Part model, mm, in its own coordinate system. A direction names the side the tool comes from. Coordinates: 2 decimals unless noted, no trailing zeros. Loops run counter-clockwise (first coordinate to the right, second up) from the corner with the lowest first, then second, coordinate; pieces in that order, holes last. Notation, with made-up numbers: (56, 6.25) -> (110, 6.25) arc R10 cw to (110, 11.25) -> close; hole circle Ø6 at (-30, 45.25). An arc over 180 degrees is marked (long way). One line per question, with ' | ' between items. Start each with the question number.
1) Cut at D-D (z = 30). List the corners of the cut face in (x, y), plus the area to 3 significant figures.
2) Two-plate mould, pull along Z, no slides. Class faces 1 (the face through (5, 5, 0)), 2 (the face through (9, 17, -9)), 3 (the face through (-0.88, 10.92, 19.98)): released by +Z, released by -Z, zero draft, split by the parting line, or undercut.
3) Drop flat-ended pins along their axis: pin 1 (12.5 mm diameter, centred on x = 0.5, z = -5, fed in from +Y); pin 2 (6 mm diameter, centred on y = 4, z = 29.5, fed in from +X); pin 3 (10 mm diameter, centred on x = 12.5, y = 3.5, fed in from +Z). Give the stop position or say it passes through.
4) Probe L1, parallel to X at y = 3.6, z = 0; L2, parallel to X at y = 13.5, z = 0; L3, parallel to Y at x = 32, z = -12. List the from-to ranges inside material, lowest first. Write a range as from..to.
5) 3-axis set-ups, long thin cutter, end or side, ignore diameter. For faces 4 (the face through (25.85, 2.46, 0.92)), 5 (the face through (-18.3, 5, -9.4)): which of +Z, -Z, +X, -X, +Y, -Y reach the whole face in a straight line?
6) Cut at A-A (x = 0). List the corners of the cut face in (y, z), plus the area to 3 significant figures.
7) Cut at B-B (z = 0). List the corners of the cut face in (x, y), plus the area to 3 significant figures.
8) Cut at C-C (y = 2.25). List the corners of the cut face in (x, z), plus the area to 3 significant figures.
from build123d import *

# Parameters (mm, degrees)
SKETCH2_R          = 4.25
CUT_EXTRUDE1_DEPTH = 10


with BuildPart() as part:
    # Sketch1 → Revolve1 (revolve)
    with BuildSketch(Plane.XY, mode=Mode.PRIVATE) as revolve1_sk:
        Polygon((4.5, 5), (12.5, 5), (12.5, 17), (20, 17), (20, 5), (40, 5), (40, 0), (4.5, 0), align=None)
    revolve(revolve1_sk.sketch.rotate(Axis((0, 0, 0), (0, 1, 0)), 90), axis=Axis((0, 0, 0), (0, 1, 0)))

    # Sketch2 → Cut-Extrude1 (cut)
    with BuildSketch(Plane.XZ):
        with Locations(Location((0, 30, 0), (0, 0, 270))):
            Circle(SKETCH2_R)
        with Locations(Location((30, 0, 0), (0, 0, 270))):
            Circle(SKETCH2_R)
        with Locations(Location((0, -30, 0), (0, 0, 270))):
            Circle(SKETCH2_R)
        with Locations(Location((-30, 0, 0), (0, 0, 270))):
            Circle(SKETCH2_R)
    extrude(amount=-CUT_EXTRUDE1_DEPTH, mode=Mode.SUBTRACT)


solid = part.part
Reported:
1) outline: (-26.46, 0) -> (-4.25, 0) -> (-4.25, 5) -> (-26.46, 5) -> close; (4.25, 0) -> (26.46, 0) -> (26.46, 5) -> (4.25, 5) -> close | area: 222 mm²
2) face 1: undercut | face 2: zero draft | face 3: split by the parting line
3) pin 1: stops at y = 5 | pin 2: stops at x = 29.96 | pin 3: stops at z = 39.29
4) L1: x = -40..-34.25, -25.75..-4.5, 4.5..25.75, 34.25..40 | L2: x = -20..-12.5, 12.5..20 | L3: y = 0..5
5) face 4: +Y, -Y | face 5: +Y
6) outline: (0, -40) -> (5, -40) -> (5, -34.25) -> (0, -34.25) -> close; (0, -25.75) -> (5, -25.75) -> (5, -20) -> (17, -20) -> (17, -12.5) -> (5, -12.5) -> (5, -4.5) -> (0, -4.5) -> close; (0, 4.5) -> (5, 4.5) -> (5, 12.5) -> (17, 12.5) -> (17, 20) -> (5, 20) -> (5, 25.75) -> (0, 25.75) -> close; (0, 34.25) -> (5, 34.25) -> (5, 40) -> (0, 40) -> close | area: 450 mm²
7) outline: (-40, 0) -> (-34.25, 0) -> (-34.25, 5) -> (-40, 5) -> close; (-25.75, 0) -> (-4.5, 0) -> (-4.5, 5) -> (-12.5, 5) -> (-12.5, 17) -> (-20, 17) -> (-20, 5) -> (-25.75, 5) -> close; (4.5, 0) -> (25.75, 0) -> (25.75, 5) -> (20, 5) -> (20, 17) -> (12.5, 17) -> (12.5, 5) -> (4.5, 5) -> close; (34.25, 0) -> (40, 0) -> (40, 5) -> (34.25, 5) -> close | area: 450 mm²
8) outline: circle Ø80 at (0, 0); hole circle Ø8.5 at (-30, 0); hole circle Ø9 at (0, 0); hole circle Ø8.5 at (0, -30); hole circle Ø8.5 at (0, 30); hole circle Ø8.5 at (30, 0) | area: 4,740 mm²
